Could you check a few things on this model? Use its own coordinates, in mm. A direction names the side the tool comes from. Coordinates: 2 decimals unless noted, no trailing zeros. Loops run counter-clockwise (first coordinate to the right, second up) from the corner with the lowest first, then second, coordinate; pieces in that order, holes last. Notation, with made-up numbers: (30, 69) -> (79, 69) arc R21 ccw to (79, 91) -> close; hole circle Ø5 at (6.5, 71.25). An arc over 180 degrees is marked (long way). One line per question, with ' | ' between items.
Autodesk Fusion 360 part; units mm, degrees
sketch "Sketch1" plane through (0, 0, 0) normal (1, 0, 0) x (0, 0, -1)
  line L0 (10, -1.9638) -> (10, -11)
  line L1 (6, -15) -> (-6, -15)
  line L2 (-10, -11) -> (-10, -1.9638)
  line L3 (-65, -40) -> (65, -40)
  line L4 (-11.5882, -1.155) -> (-65, -40)
  line L5 (65, -40) -> (11.5882, -1.155)
  arc A0 (-10, -11) -> (-6, -15) centre (-6, -11) ccw
  arc A1 (6, -15) -> (10, -11) centre (6, -11) ccw
  arc A2 (-10, -1.9638) -> (-11.5882, -1.155) centre (-11, -1.9638) ccw
  arc A3 (11.5882, -1.155) -> (10, -1.9638) centre (11, -1.9638) ccw
  point P0 (10, 0)
  dimension "d136" = 20
  dimension "d137" = 10
  dimension "d138" = 65
  dimension "d139" = 4
  dimension "d140" = 4
  dimension "d141" = 1
  dimension "d142" = 1
extrude "Extrude1" add sketch "Sketch1" along normal blind 3.5
equation "d138 = ( 130 / 2 ) * 1 mm"
Q1. Imagine slicing it at C-C on z = 15. Write out the boundary of the cut face in (x, y), plus the area to 3 significant figures.
Values follow:
outline: (0, -40) -> (3.5, -40) -> (3.5, -3.64) -> (0, -3.64) -> close | area: 127 mm2
Q2. For pin 1 (2 mm diameter, centred on x = 1.5, y = -30.5, fed in from +Z); pin 2 (1 mm diameter, centred on x = 1, y = -5, fed in from -Z), each with a flat end and sliding along its axis, tell me the tip position at first contact or that it passes through.
Values follow:
pin 1: stops at z = 53.31 | pin 2: stops at z = -17.56
Q3. Please list where these lines run through material, in increasing order: L1, parallel to Z at x = 1.65, y = -8.5; L2, parallel to Y at x = 2.4, z = 1; L3, parallel to Z at x = 2.6, y = -3. Write a range as [from, to].
Values follow:
L1: z = [-21.69, -10], [10, 21.69] | L2: y = [-40, -15] | L3: z = [-14.13, -10], [10, 14.13]
Q4. Imagine slicing it at D-D on y = -31.5. Write out the boundary of the cut face in (x, z).
Values follow:
outline: (0, -53.31) -> (3.5, -53.31) -> (3.5, 53.31) -> (0, 53.31) -> close
Q5. Imagine slicing it at A-A on y = -13.5. Write out the boundary of the cut face in (x, z), plus the area to 3 significant figures.
Values follow:
outline: (0, -28.56) -> (3.5, -28.56) -> (3.5, -9.12) -> (0, -9.12) -> close; (0, 9.12) -> (3.5, 9.12) -> (3.5, 28.56) -> (0, 28.56) -> close | area: 136 mm2
Q6. Imagine slicing it at B-B on x = 1.3. Write out the boundary of the cut face in (y, z) (3 decimals), plus the area to 3 significant figures.
Values follow:
outline: (-40, -65) -> (-1.155, -11.588) arc R1 ccw to (-1.964, -10) -> (-11, -10) arc R4 cw to (-15, -6) -> (-15, 6) arc R4 cw to (-11, 10) -> (-1.964, 10) arc R1 ccw to (-1.155, 11.588) -> (-40, 65) -> close | area: 2,710 mm2
Q7. We'd pull the mould along Z, two halves only. Please class faces 3 (the face through (2, -40, 1)), 4 (the face through (2, -15, 0)), 5 (the face through (1.726, -20.306, 37.92)), 6 (the face through (1.73, -20.85, -38.67)): released by +Z, released by -Z, zero draft, split by the parting line, or undercut.
Values follow:
face 3: zero draft | face 4: undercut | face 5: released by +Z | face 6: released by -Z
Q8. For faces 1 (the face through (1.726, -13.797, -8.859)), 2 (the face through (3.5, -25, 1)), which set-ups out of +Z, -Z, +X, -X, +Y, -Y let a thin tool reach every point of the face, with its end or its side?
Values follow:
face 1: +X, -X, +Y | face 2: +Z, -Z, +X, +Y, -Y
